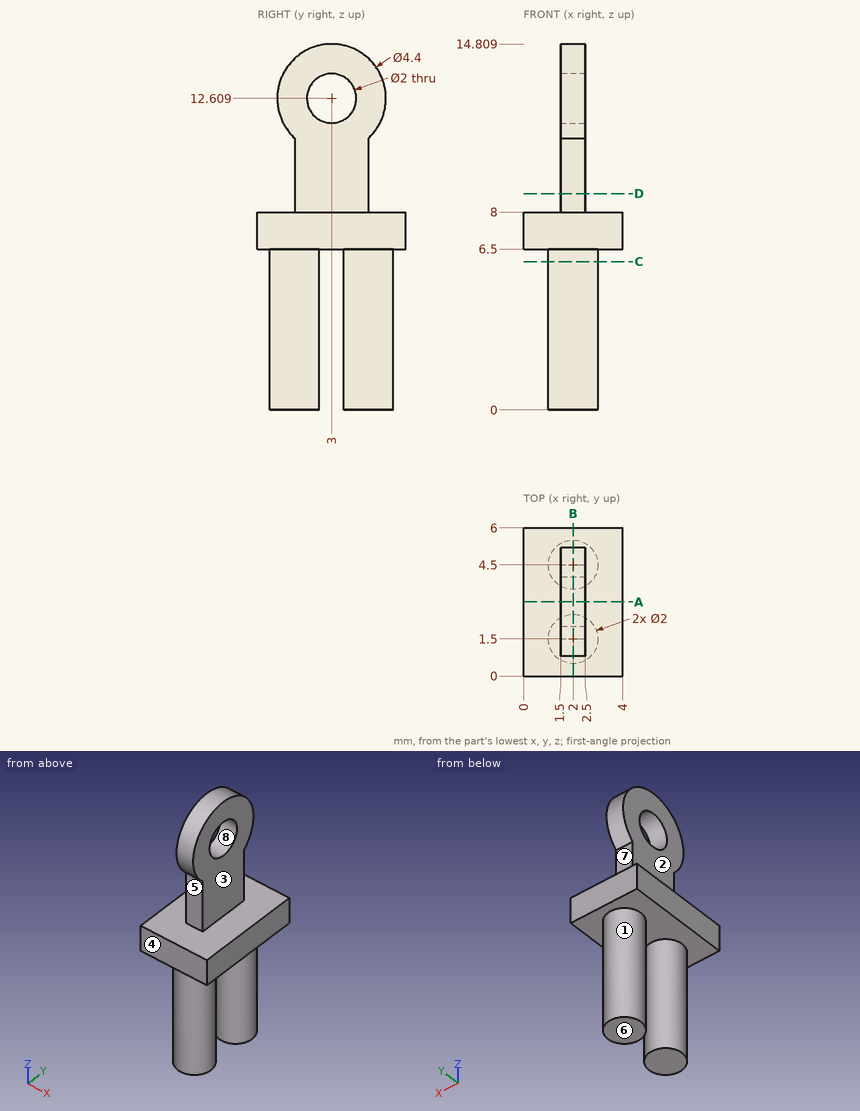
For this review, use the dimensioned drawing (mm, ordinates from the lowest corner) and the shaded views. A direction names the side the tool comes from. Round coordinates to 2 decimals unless told otherwise and drop trailing zeros. Write each loop counter-clockwise with the first axis right and the second up, starting at its lowest first coordinate (ties: lowest second). Pieces come first, ordered by that corner, then holes. Notation, with made-up numbers: M -33.75,-5.75 L -14.75,-5.75 A19 ccw -14.75,0.25 Z; hole C 14.5,78 d9. An arc over 180 degrees is marked long. Write item = value, one per line. Start each with the question number.
(1) We need section B-B (x = 2). Give the boundary of the cut face in (y, z).
(2) We need section D-D (z = 8.75). Give the boundary of the cut face in (x, y).
(3) We need section C-C (z = 6). Give the boundary of the cut face in (x, y).
(4) The part is to be moulded in two halves that separate along Y. For the marked faces 6, 7 and 8, say which applies: +Y half, -Y half, draft (parallel to the pull), parting line (faces both ways), or undercut.
(5) Clearance check with flat-ended pins moving along their axes: pin 1 Ø1.8 at (y, z) = (3, 12.61) entering from -X; pin 2 Ø2 at (y, z) = (1, 9.5) entering from +X; pin 3 Ø3 at (y, z) = (4.5, 3.5) entering from -X; pin 4 Ø0.8 at (x, z) = (2, 9) entering from +Y. State where each tip first meets the part, or that it passes through.
(6) For the marked faces 1, 2, 3, 4 and 5, list the 3-axis set-ups (+Z, -Z, +X, -X, +Y, -Y) from which the entire face can be reached by the end or side of a thin tool; tool diameter is ignored.
(7) We need section A-A (y = 3). Give the boundary of the cut face in (x, z).
(8) For line 1 along X through (y, z) = (1.55, 0.75); line 2 along Y through (x, z) = (2.45, 4); line 3 along Z through (x, y) = (3.2, 1.35), list the stretches that pass through material, from the lowest coordinate up.
Results found:
q1.outline = M 0,6.5 L 0.5,6.5 L 0.5,0 L 2.5,0 L 2.5,6.5 L 3.5,6.5 L 3.5,0 L 5.5,0 L 5.5,6.5 L 6,6.5 L 6,8 L 4.5,8 L 4.5,11 A2.2 ccw long 1.5,11 L 1.5,8 L 0,8 Z; hole C 3,12.61 d2
q2.outline = M 1.5,1.5 L 2.5,1.5 L 2.5,4.5 L 1.5,4.5 Z
q3.outline = C 2,1.5 d2; C 2,4.5 d2
q4.face_6 = draft
q4.face_7 = +Y half
q4.face_8 = undercut
q5.pin_1 = through
q5.pin_2 = 2.5
q5.pin_3 = 1
q5.pin_4 = 4.5
q6.face_1 = -Z
q6.face_2 = +Z, -X, +Y, -Y
q6.face_3 = +Z, +X, +Y, -Y
q6.face_4 = +Z, -Z, +X, -X, -Y
q6.face_5 = +X, -X, -Y
q7.outline = M 0,6.5 L 4,6.5 L 4,8 L 2.5,8 L 2.5,11.61 L 1.5,11.61 L 1.5,8 L 0,8 Z; M 1.5,13.61 L 2.5,13.61 L 2.5,14.81 L 1.5,14.81 Z
q8.line_1 = 1 to 3
q8.line_2 = 0.61 to 2.39, 3.61 to 5.39
q8.line_3 = 6.5 to 8
